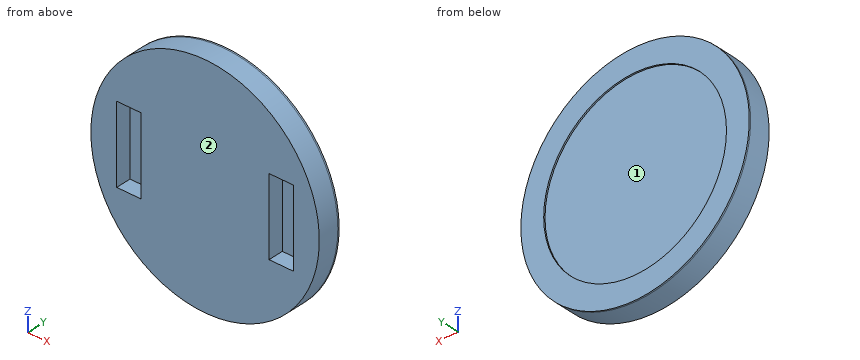
Autodesk Inventor part; units mm, degrees
ref_plane "YZ Plane" through (0, 0, 0) normal (1, 0, 0) x (0, 1, 0)
ref_plane "XZ Plane" through (0, 0, 0) normal (0, 1, 0) x (-1, 0, 0)
ref_plane "XY Plane" through (0, 0, 0) normal (0, 0, 1) x (1, 0, 0)
sketch "Sketch1" plane through (0, 0, 0) normal (0, 1, 0) x (-1, 0, 0)
  circle A0 centre (0, 0) radius 15
  dimension "d0" = 30
extrude "Extrusion1" add sketch "Sketch1" against normal blind 2.8
sketch "Sketch2" plane through (0, 0, 0) normal (0, 1, 0) x (1, 0, 0)
  line L0 (7.5, -7.5) -> (-7.5, -7.5)
  line L1 (-7.5, -7.5) -> (-7.5, 7.5)
  line L2 (-7.5, 7.5) -> (7.5, 7.5)
  line L3 (7.5, 7.5) -> (7.5, -7.5)
  line L4 (7.5, -7.5) -> (-7.5, 7.5) construction
  line L5 (-7.5, -7.5) -> (7.5, 7.5) construction
  circle A0 centre (0, 0) radius 12
  circle A1 centre (0, 0) radius 15
  dimension "d3" = 15
  dimension "d4" = 15
  dimension "d13" = 3
extrude "Extrusion2" add sketch "Sketch2" along normal blind 0.2 contours A1
sketch "Sketch3" plane through (0, -2.8, 0) normal (0, -1, 0) x (1, 0, 0)
  line L0 (10, 0) -> (-10, 0) construction
  line L1 (-11.6, -5.1) -> (-8.4, -5.1)
  line L2 (-8.4, -5.1) -> (-8.4, 5.1)
  line L3 (-8.4, 5.1) -> (-11.6, 5.1)
  line L4 (-11.6, 5.1) -> (-11.6, -5.1)
  line L5 (-11.6, -5.1) -> (-8.4, 5.1) construction
  line L6 (-8.4, -5.1) -> (-11.6, 5.1) construction
  line L7 (0, -15) -> (0, 15) construction
  circle A0 centre (0, 0) radius 15 construction
  line L8 (11.6, -5.1) -> (8.4, -5.1)
  line L9 (8.4, -5.1) -> (8.4, 5.1)
  line L10 (8.4, 5.1) -> (11.6, 5.1)
  line L11 (11.6, 5.1) -> (11.6, -5.1)
  line L12 (11.6, -5.1) -> (8.4, 5.1) construction
  line L13 (8.4, -5.1) -> (11.6, 5.1) construction
  dimension "d14" = 20
  dimension "d15" = 3.2
  dimension "d16" = 10.2
extrude "Extrusion3" cut sketch "Sketch3" against normal blind 2
extrude "Extrusion4" [suppressed]
extrude "Extrusion5" [suppressed]
properties part number "Tag"
CAD build for the part. Positions are in the model's coordinates, mm. Face numbers are marked on the shaded views. Round coordinates to 2 decimals unless told otherwise and drop trailing zeros. Write each loop counter-clockwise with the first axis right and the second up, starting at its lowest first coordinate (ties: lowest second). Pieces come first, ordered by that corner, then holes. Notation, with made-up numbers: M 38,71 L 47,71 A15 cw 47,93 Z; hole C 70.5,74 d1. An arc over 180 degrees is marked long. Use a Markdown table: item, result. Add a question column.
1. Drill centre lines: probe 1 along X at (y, z) = (0.15, 0); probe 2 along X at (y, z) = (-1.7, 1). Where is each one in solid material? Low to high.
2. Flat gauge pins, fed straight in: P1, Ø1.6, axis at y = -1.5, z = -1, coming from the -X side; P2, Ø1, axis at x = -10.5, y = -1.5, coming from the +Z side; P3, Ø1.6, axis at y = -1.5, z = 2, coming from the +X side. Where does each tip first touch, or does it go through?
3. Slice it at B-B on x = 0. Give the cut face in (y, z).
4. Slice it at D-D on z = 0. Give the cut face in (x, y).
5. Pull direction X, two halves, no side cores. Call the marked faces 1 and 2: released by +X, released by -X, zero draft, split by the parting line, or undercut.
6. Slice it at A-A on y = -1.9. Give the cut face in (x, z).
7. Slice it at C-C on z = 11.25. Give the cut face in (x, y), then the cut area to 3 significant figures.
Reply:
| question | item | result |
|---|---|---|
| 1 | probe 1 | x = -15 to -12, 12 to 15 |
| 1 | probe 2 | x = -14.97 to -11.6, -8.4 to 8.4, 11.6 to 14.97 |
| 2 | P1 | stops at x = -15 |
| 2 | P2 | stops at z = 11.18 |
| 2 | P3 | stops at x = 14.95 |
| 3 | outline | M -2.8,-15 L 0.2,-15 L 0.2,-12 L 0,-12 L 0,12 L 0.2,12 L 0.2,15 L -2.8,15 Z |
| 4 | outline | M -15,-2.8 L -11.6,-2.8 L -11.6,-0.8 L -8.4,-0.8 L -8.4,-2.8 L 8.4,-2.8 L 8.4,-0.8 L 11.6,-0.8 L 11.6,-2.8 L 15,-2.8 L 15,0.2 L 12,0.2 L 12,0 L -12,0 L -12,0.2 L -15,0.2 Z |
| 5 | face 1 | undercut |
| 5 | face 2 | zero draft |
| 6 | outline | C 0,0 d30; hole M -11.6,-5.1 L -8.4,-5.1 L -8.4,5.1 L -11.6,5.1 Z; hole M 8.4,-5.1 L 11.6,-5.1 L 11.6,5.1 L 8.4,5.1 Z |
| 7 | outline | M -9.92,-2.8 L 9.92,-2.8 L 9.92,0.2 L 4.18,0.2 L 4.18,0 L -4.18,0 L -4.18,0.2 L -9.92,0.2 Z |
| 7 | area | 57.9 mm^2 |
